Part print with two shaded views. Sizes in mm from the minimum x, y, z corner. A direction names the side the tool comes from. Give positions to 0.01 mm unless a question says otherwise; leave off trailing zeros. Order: outer loops, then holes, each group sorted by start corner. A loop starts at its lowest first (then second) coordinate and runs counter-clockwise, first axis right, second up. Notation, with made-up numbers: (35.5, 86) -> (42.5, 86) arc R17 ccw to (42.5, 102) -> close; hole circle Ø3 at (29.25, 52). An arc over 180 degrees is marked (long way). Write item = value, one per line. Start each with the question number.
Item 1: Band-saw the part on D-D on y = 22.5. Write the cut outline in (x, z), plus the area to 3 significant figures.
Item 2: Band-saw the part on C-C on x = 39. Write the cut outline in (y, z), plus the area to 3 significant figures.
Item 3: Band-saw the part on A-A on z = 11.25. Write the cut outline in (x, y), plus the area to 3 significant figures.
Item 4: Drill centre lines: line 1 along X through (y, z) = (22.5, 19); line 2 along Z through (x, y) = (33.5, 23). Where is each one in solid material? Low to high.
Item 5: Band-saw the part on B-B on y = 19.5. Write the cut outline in (x, z), plus the area to 3 significant figures.
Item 6: Tool access for the marked faces 1, 2 and 3: list every direction of +Z, -Z, +X, -X, +Y, -Y with a clear straight run to the whole face (end or side of a thin tool).
Item 7: Flat gauge pins, fed straight in: P1, Ø5, axis at y = 2.5, z = 13, coming from the +X side; P2, Ø4, axis at x = 14.5, y = 13, coming from the +Z side; P3, Ø2, axis at y = 9.5, z = 7.5, coming from the -X side. Where does each tip first touch, or does it go through?
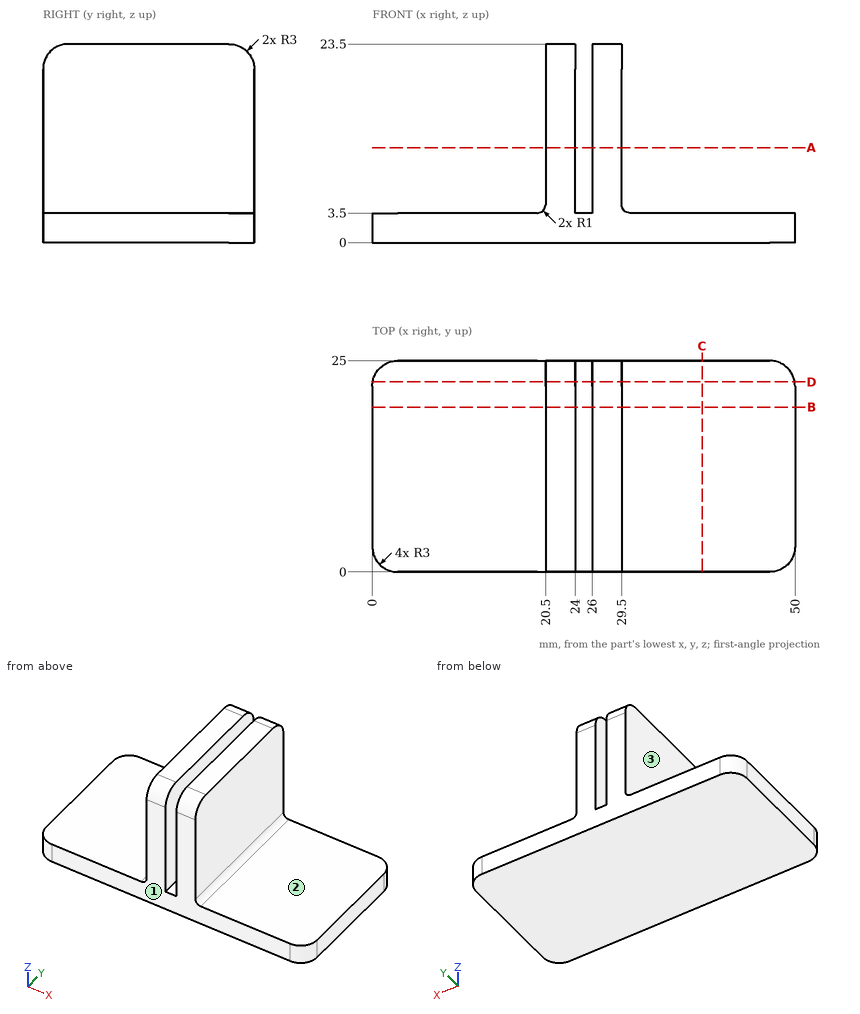
Values found:
q1.outline = (0.04, 0) -> (49.96, 0) -> (49.96, 3.5) -> (30.5, 3.5) arc R1 cw to (29.5, 4.5) -> (29.5, 23.46) -> (26, 23.46) -> (26, 3.5) -> (24, 3.5) -> (24, 23.46) -> (20.5, 23.46) -> (20.5, 4.5) arc R1 cw to (19.5, 3.5) -> (0.04, 3.5) -> close
q1.area = 315 mm^2
q2.outline = (0, 0) -> (25, 0) -> (25, 3.5) -> (0, 3.5) -> close
q2.area = 87.5 mm^2
q3.outline = (20.5, 0) -> (24, 0) -> (24, 25) -> (20.5, 25) -> close; (26, 0) -> (29.5, 0) -> (29.5, 25) -> (26, 25) -> close
q3.area = 175 mm^2
q4.line_1 = 20.5 to 24, 26 to 29.5
q4.line_2 = 0 to 3.5
q5.outline = (0, 0) -> (50, 0) -> (50, 3.5) -> (30.5, 3.5) arc R1 cw to (29.5, 4.5) -> (29.5, 23.5) -> (26, 23.5) -> (26, 3.5) -> (24, 3.5) -> (24, 23.5) -> (20.5, 23.5) -> (20.5, 4.5) arc R1 cw to (19.5, 3.5) -> (0, 3.5) -> close
q5.area = 315 mm^2
q6.face_1 = +Z, -Z, +X, -X, -Y
q6.face_2 = +Z, +X, +Y, -Y
q6.face_3 = +Z, -X, +Y, -Y
q7.P1 = 29.5
q7.P2 = 3.5
q7.P3 = 20.5
